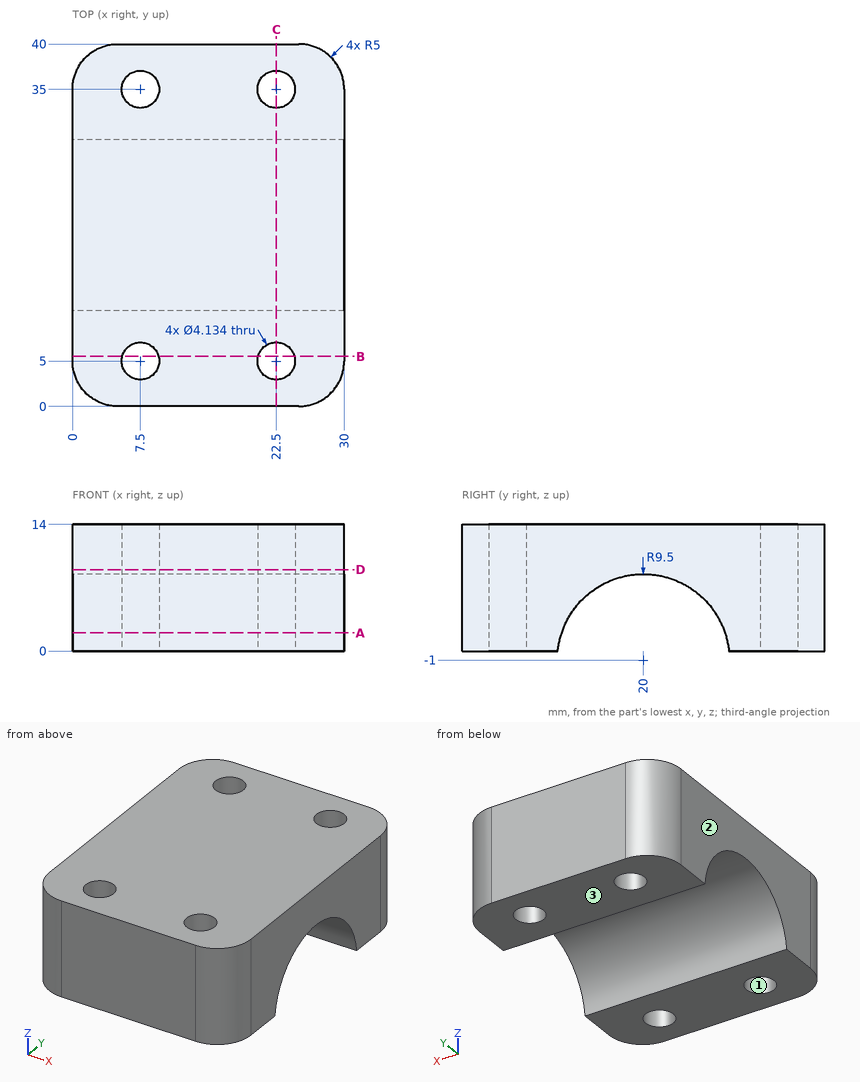
For this review, use the dimensioned drawing (mm, ordinates from the lowest corner) and the shaded views. Round coordinates to 2 decimals unless told otherwise and drop trailing zeros. Write each loop counter-clockwise with the first axis right and the second up, starting at its lowest first coordinate (ties: lowest second). Pieces come first, ordered by that corner, then holes. Notation, with made-up numbers: (23.5, -7) -> (82.5, -7) arc R25 ccw to (82.5, 6) -> close; hole circle Ø11 at (46.5, 52.5). An arc over 180 degrees is marked (long way). Use CSV: the item, a comma, the result in double quotes.
(1) Consider section B-B, the plane y = 5.5. Give the boundary of the cut face in (x, z), plus the area to 3 significant figures.
Computed values:
outline,"(0, 0) -> (5.49, 0) -> (5.49, 14) -> (0, 14) -> close; (9.51, 0) -> (20.49, 0) -> (20.49, 14) -> (9.51, 14) -> close; (24.51, 0) -> (30, 0) -> (30, 14) -> (24.51, 14) -> close"
area,"308 mm²"
(2) Consider section D-D, the plane z = 9. Give the boundary of the cut face in (x, y).
Computed values:
outline,"(0, 5) arc R5 ccw to (5, 0) -> (25, 0) arc R5 ccw to (30, 5) -> (30, 35) arc R5 ccw to (25, 40) -> (5, 40) arc R5 ccw to (0, 35) -> close; hole circle Ø4.13 at (7.5, 5); hole circle Ø4.13 at (7.5, 35); hole circle Ø4.13 at (22.5, 5); hole circle Ø4.13 at (22.5, 35)"
(3) Consider section A-A, the plane z = 2. Give the boundary of the cut face in (x, y).
Computed values:
outline,"(0, 5) arc R5 ccw to (5, 0) -> (25, 0) arc R5 ccw to (30, 5) -> (30, 10.99) -> (0, 10.99) -> close; (0, 29.01) -> (30, 29.01) -> (30, 35) arc R5 ccw to (25, 40) -> (5, 40) arc R5 ccw to (0, 35) -> close; hole circle Ø4.13 at (7.5, 5); hole circle Ø4.13 at (7.5, 35); hole circle Ø4.13 at (22.5, 5); hole circle Ø4.13 at (22.5, 35)"
(4) Draft analysis for pull direction X (two halves, no side actions). For the marked faces 1, 2 and 3, state which applies: +X half, -X half, draft (parallel to the pull), parting line (faces both ways), or undercut.
Computed values:
face 1,"undercut"
face 2,"-X half"
face 3,"draft"
(5) Clearance check with a flat-ended pin moving along its axis: P1, Ø10, axis at x = 18.5, y = 18.5, coming from the -Z side. State where the tip first meets the part, or that it passes through.
Computed values:
P1,"z = 5.93"
(6) Consider section C-C, the plane x = 22.5. Give the boundary of the cut face in (y, z), plus the area to 3 significant figures.
Computed values:
outline,"(0, 0) -> (2.93, 0) -> (2.93, 14) -> (0, 14) -> close; (7.07, 0) -> (10.55, 0) arc R9.5 cw to (29.45, 0) -> (32.93, 0) -> (32.93, 14) -> (7.07, 14) -> close; (37.07, 0) -> (40, 0) -> (40, 14) -> (37.07, 14) -> close"
area,"321 mm²"
(7) To check wall thickness, follow L1, parallel to X at y = 5, z = 4.25; L2, parallel to Y at x = 21, z = 11.75; L3, parallel to Y at x = 7.5, z = 3. State the ranges of each line that lie inside material, in increasing order. Write a range as [from, to].
Computed values:
L1,"[0, 5.43], [9.57, 20.43], [24.57, 30]"
L2,"[0, 3.58], [6.42, 33.58], [36.42, 40]"
L3,"[0, 2.93], [7.07, 11.38], [28.62, 32.93], [37.07, 40]"
